```python
from build123d import *

# Parameters (mm, degrees)
F0_W     = 59.1693818569
F0_H     = 40.4018647969
F1_DEPTH = 38.1


with BuildPart() as f1:
    # F0 (on Top) → F1 (new body, symmetric)
    with BuildSketch(Plane.XY):
        with Locations((29.5846909285, 20.2009323984)):
            Rectangle(F0_W, F0_H)
        Polygon((59.1693818569, 0), (0, 0), (0, -52.4184517562), (71.0263326764, -52.4184517562), (71.0263326764, 0), align=None)
    extrude(amount=F1_DEPTH, both=True)


solid = f1.part
```
Model file for the job. Use its own axes, mm. A direction names the side the tool comes from. Coordinates: 2 decimals unless noted, no trailing zeros. Loops run counter-clockwise (first coordinate to the right, second up) from the corner with the lowest first, then second, coordinate; pieces in that order, holes last. Notation, with made-up numbers: (43.5, 80) -> (47.5, 80) arc R37 ccw to (47.5, 117) -> close; hole circle Ø10 at (-28, 79.25). An arc over 180 degrees is marked (long way). Answer as a JSON object with one key per item and string values.
Q1. Flat gauge pins, fed straight in: P1, Ø12, axis at y = 17, z = 4.5, coming from the +X side; P2, Ø3.5, axis at x = 67, z = 1, coming from the +Y side. Where does each tip first touch, or does it go through?
Report:
{"P1": "stops at x = 59.17", "P2": "stops at y = 0"}
Q2. Cut at A-A (z = 33). List the corners of the cut face in (x, y), and give its area (3 significant figures).
Report:
{"outline": "(0, -52.42) -> (71.03, -52.42) -> (71.03, 0) -> (59.17, 0) -> (59.17, 40.4) -> (0, 40.4) -> close", "area": "6,110 mm2"}
Q3. 3-axis set-ups, long thin cutter, end or side, ignore diameter. For faces 1 (the flat face through (65, 0, 1)), 2 (the flat face through (35, -5, -38.1)): which of +Z, -Z, +X, -X, +Y, -Y reach the whole face in a straight line?
Report:
{"face 1": "+Z, -Z, +X, +Y", "face 2": "-Z, +X, -X, +Y, -Y"}
Q4. Probe probe 1 along Y at (x, z) = (61, 23.5); probe 2 along X at (y, z) = (10, -10). List the from-to ranges inside material, lowest first.
Report:
{"probe 1": "y = -52.42 to 0", "probe 2": "x = 0 to 59.17"}
Q5. Cut at B-B (y = 2.5). List the corners of the cut face in (x, z).
Report:
{"outline": "(0, -38.1) -> (59.17, -38.1) -> (59.17, 38.1) -> (0, 38.1) -> close"}
